Read the model definition and answer for the solid it produces. Units are mm, in the model's axes. A direction names the side the tool comes from. Round coordinates to 2 decimals unless told otherwise and drop trailing zeros. Order: outer loops, then holes, each group sorted by start corner. A loop starts at its lowest first (then second) coordinate and runs counter-clockwise, first axis right, second up.
from build123d import *

# Parameters (mm, degrees)
SKETCH3_W           = 20
SKETCH3_H           = 20
SKETCH3_R           = 2.1
BOSS_EXTRUDE1_DEPTH = 50
CUT_EXTRUDE1_START  = -1
CUT_EXTRUDE1_DEPTH  = 52
CIRPATTERN1_COUNT   = 4
CHAMFER2_SIZE       = 1.7
FILLET1_R           = 0.14


with BuildPart() as part:
    # Sketch3 → Boss-Extrude1 (new body)
    with BuildSketch(Plane(origin=(0, 0, 0), x_dir=(1, 0, 0), z_dir=(0, 1, 0))):
        Rectangle(SKETCH3_W, SKETCH3_H)
        Circle(SKETCH3_R, mode=Mode.SUBTRACT)
    extrude(amount=BOSS_EXTRUDE1_DEPTH)

    # Sketch4 → Cut-Extrude1 (cut)
    with BuildSketch(Plane(origin=(0, 0, 0), x_dir=(1, 0, 0), z_dir=(0, 1, 0)).offset(CUT_EXTRUDE1_START)):
        Polygon((-3.1, 10), (-3.1, 8.2), (-5.5, 8.2), (-5.5, 6.560660172), (-2.839339828, 3.9), (-0.15, 3.9), (0, 3.75), (0.15, 3.9), (2.839339828, 3.9), (5.5, 6.560660172), (5.5, 8.2), (3.1, 8.2), (3.1, 10), align=None)
    cut_extrude1 = extrude(amount=CUT_EXTRUDE1_DEPTH, mode=Mode.SUBTRACT)

    # CirPattern1: Cut-Extrude1 ×4 about axis
    cirpattern1_axis = Axis((0, 0, 0), (0, 1, 0))
    for i in range(1, CIRPATTERN1_COUNT):
        add(cut_extrude1.rotate(cirpattern1_axis, i * 360 / CIRPATTERN1_COUNT), mode=Mode.SUBTRACT)

    # Chamfer2
    chamfer2_edges = [part.edges().sort_by_distance(p)[0] for p in [
        (-3.1, 25, 10),
        (3.1, 25, 10),
        (-10, 25, -3.1),
        (-10, 25, 3.1),
        (10, 25, 3.1),
        (10, 25, -3.1),
        (3.1, 25, -10),
        (-3.1, 25, -10),
    ]]
    chamfer(chamfer2_edges, length=CHAMFER2_SIZE)

    # Fillet1
    fillet1_edges = [part.edges().sort_by_distance(p)[0] for p in [
        (10, 25, 10),
        (-10, 25, 10),
        (-10, 25, -10),
        (10, 25, -10),
    ]]
    fillet(fillet1_edges, radius=FILLET1_R)


solid = part.part
Q1. For faces 1 (the face through (-9.2, 24.7, -4)), 2 (the face through (3.9, 25, -2)), 3 (the face through (5.21, 24.65, 4.15)), determine the directions among +Z, -Z, +X, -X, +Y, -Y from which every point of the face is accessible in a straight line to the end or side of a thin tool.
Outcome:
face 1: -X, +Y, -Y
face 2: +X, +Y, -Y
face 3: +Y, -Y
Q2. For a pull along X with two mould halves and no side action, classify faces 4 (the face through (3.9, 25, 1)), 5 (the face through (-10, 25, 7)), 6 (the face through (4, 25, 8.2)), 7 (the face through (7, 25, 10)) as released by +X, released by -X, zero draft, split by the parting line, or undercut.
Outcome:
face 4: released by +X
face 5: released by -X
face 6: undercut
face 7: zero draft
Q3. A cutting plane is placed at A-A, the plane z = -1. Give the vertices of the cut face in (x, y), plus the area to 3 significant figures.
Outcome:
outline: (-3.9, 0) - (-1.85, 0) - (-1.85, 50) - (-3.9, 50) - close; (1.85, 0) - (3.9, 0) - (3.9, 50) - (1.85, 50) - close
area: 205 mm2
Q4. Straight lines are drawn through the part: probe 1 along X at (y, z) = (13, -5); probe 2 along X at (y, z) = (7, -8.25); probe 3 along X at (y, z) = (37.5, 8). For each, find the intervals that lie inside material, in ascending order.
Outcome:
probe 1: x = -10 to -8.2, -6.06 to -3.94, 3.94 to 6.06, 8.2 to 10
probe 2: x = -10 to -3.1, 3.1 to 10
probe 3: x = -10 to -5.5, 5.5 to 10
Q5. Flat-ended cylindrical pins translate along their axes: pin 1 (1.2 mm diameter, centred on x = -3.5, y = 37, fed in from +Z); pin 2 (1 mm diameter, centred on x = -3, z = -5.5, fed in from -Y); pin 3 (0.7 mm diameter, centred on y = 30.5, z = -4, fed in from -X); pin 4 (0.8 mm diameter, centred on x = -1.5, y = 22, fed in from -Z). Find the tip coordinate at first contact, or state that the pin passes through.
Outcome:
pin 1: stops at z = 9.3
pin 2: passes through
pin 3: stops at x = -9.55
pin 4: stops at z = -3.9
